Input: part model. Units: mm. Frame: model coordinates. A direction names the side the tool comes from. Coordinates: 2 decimals unless noted, no trailing zeros. Loops run counter-clockwise (first coordinate to the right, second up) from the corner with the lowest first, then second, coordinate; pieces in that order, holes last.
(1) Set-up query: faces 1 (the face through (18.623, -12.325, -21.08)), 2 (the face through (5.284, -12.325, 26.336)), 3 (the face through (-1, 0, 0)), 4 (the face through (-18.623, -12.325, 21.08)), 5 (the face through (8.59, -12.32, -25.45)). Return all of +Z, -Z, +X, -X, +Y, -Y with unobstructed straight access to the full face (end or side cutting, diameter ignored); none if empty.
(2) Line query: L1, parallel to X at y = -11.5, z = 27; L2, parallel to X at y = -12, z = -15.5; L3, parallel to X at y = -20.75, z = -18.5. Output: solid intervals per line, ascending.
(3) Section A-A, the plane x = 7.5. Return loops of the section in (y, z).
(4) Mould query, pull axis Z, two halves, no side actions, for faces 6 (the face through (2.09, -12.325, -32.412)), 7 (the face through (-19.374, -12.325, 23.668)), 8 (the face through (-4.945, -12.325, 30.184)). Classes: released by +Z, released by -Z, zero draft, split by the parting line, or undercut.
(5) Contact query for flat-ended pins moving along their axis: P1, Ø3, axis at y = -8, z = 22.5, coming from the -X side; P2, Ø1.5, axis at y = -10.5, z = -12, coming from the +X side; P3, Ø1, axis at y = -10, z = 20, coming from the -X side. Output: stop coordinate, or through.
```python
from build123d import *

# Parameters (mm, degrees)
F1_DEPTH = 25
F2_DEPTH = 25
F3_COUNT = 12


with BuildPart() as f1:
    # F0 (on Front) → F1 (new body)
    with BuildSketch(Plane.XZ):
        with BuildLine():
            ThreePointArc((-5.5845651505, 26.2735435815), (-16.9038789635, -20.874514036), (26.8605, 0))
            ThreePointArc((26.8605, 0), (19.7242535187, 18.2329450002), (2.1074028217, 26.7777017983))
            ThreePointArc((2.1074028217, 26.7777017983), (-1.7567607527, 26.8029896077), (-5.5845651505, 26.2735435815))
        make_face()
        with BuildLine():
            ThreePointArc((4.0227100868, 11.3209239617), (9.8151901419, 6.9287486797), (12.0143878658, 0))
            ThreePointArc((12.0143878658, 0), (9.8151901419, -6.9287486797), (4.0227100868, -11.3209239617))
            ThreePointArc((4.0227100868, -11.3209239617), (0, -12.0143878658), (-4.0227100868, -11.3209239617))
            ThreePointArc((-4.0227100868, -11.3209239617), (-12.0143878658, 0), (-4.0227100868, 11.3209239617))
            ThreePointArc((-4.0227100868, 11.3209239617), (0, 12.0143878658), (4.0227100868, 11.3209239617))
        make_face(mode=Mode.SUBTRACT)
        with BuildLine():
            Line((4.0227100868, -11.3209239617), (4.0227100868, 11.3209239617))
            ThreePointArc((4.0227100868, 11.3209239617), (0, 12.0143878658), (-4.0227100868, 11.3209239617))
            Line((-4.0227100868, 11.3209239617), (-4.0227100868, -11.3209239617))
            ThreePointArc((-4.0227100868, -11.3209239617), (0, -12.0143878658), (4.0227100868, -11.3209239617))
        make_face()
    extrude(amount=F1_DEPTH)

    # F0 (on Front) → F2 (join)
    with BuildSketch(Plane.XZ):
        with BuildLine():
            ThreePointArc((-5.5845651505, 26.2735435815), (-1.7567607527, 26.8029896077), (2.1074028217, 26.7777017983))
            ThreePointArc((2.1074028217, 26.7777017983), (1.945127207, 28.0438038567), (1.6670221767, 29.2895989399))
            ThreePointArc((1.6670221767, 29.2895989399), (0.973127852, 30.5538872836), (0.1667310445, 31.7495622137))
            ThreePointArc((0.1667310445, 31.7495622137), (-2.1242907577, 32.4104138918), (-4.3094540977, 31.4561775392))
            ThreePointArc((-4.3094540977, 31.4561775392), (-4.952885173, 30.1654758692), (-5.4758203921, 28.8214323036))
            ThreePointArc((-5.4758203921, 28.8214323036), (-5.5889373069, 27.5499951794), (-5.5845651505, 26.2735435815))
        make_face()
    extrude(amount=F2_DEPTH)

    # F3: F1 ×12 about axis
    f3_axis = Axis((0, 0, 0), (0, 1, 0))


with BuildPart() as f1_1:
    add(f1.part)
    for i in range(1, F3_COUNT):
        add(f1.part.rotate(f3_axis, i * 360 / F3_COUNT))


solid = f1_1.part
```
Report:
1. face 1: +X, +Y, -Y
1. face 2: +Z, +Y, -Y
1. face 3: +Z, -Z, +X, -X, +Y
1. face 4: -X, +Y, -Y
1. face 5: -Z, +Y, -Y
2. L1: x = -18.05 to -14.53, -5.6 to 2.09, 9.16 to 16.06
2. L2: x = -27.48 to 21.94, 22.78 to 28.24
2. L3: x = -26.64 to -20.85, -19.47 to 19.47
3. outline: (-25, -25.79) - (0, -25.79) - (0, 25.79) - (-25, 25.79) - close
4. face 6: released by -Z
4. face 7: undercut
4. face 8: released by +Z
5. P1: stops at x = -19.41
5. P2: stops at x = 29.49
5. P3: stops at x = -18.47
